Geometry check sheet. Reference: the model listing, model coordinates, mm. Face numbers are marked on the shaded views. A direction names the side the tool comes from. Coordinates: 2 decimals unless noted, no trailing zeros. Order: outer loops, then holes, each group sorted by start corner. A loop starts at its lowest first (then second) coordinate and runs counter-clockwise, first axis right, second up. Notation, with made-up numbers: (42, 19) -> (63, 19) arc R28 cw to (63, 52) -> close; hole circle Ø6 at (50.25, 70). An arc over 180 degrees is marked (long way). Answer as CSV lines item,"result". Start each with the question number.
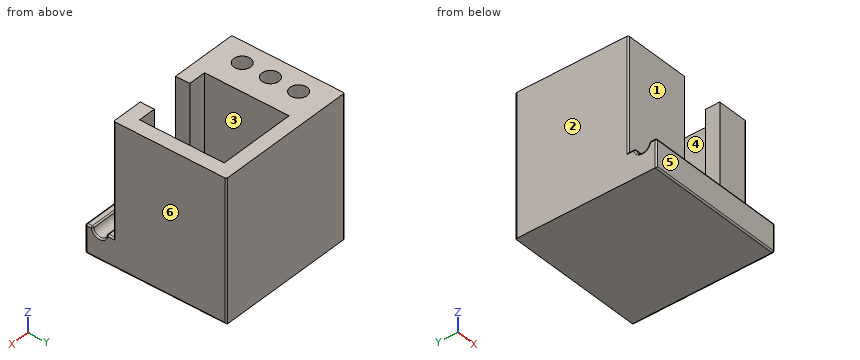
from build123d import *

# Parameters (mm, degrees)
F0_W     = 100
F0_H     = 100
F1_DEPTH = 100
F2_W     = 100
F2_H     = 20
F3_DEPTH = 80
F4_W     = 30
F4_H     = 10
F5_DEPTH = 80
F6_R     = 6
F7_DEPTH = 80
F9_DEPTH = 100
F10_R    = 1


with BuildPart() as f1:
    # F0 (on Top) → F1 (new body)
    with BuildSketch(Plane.XY):
        Rectangle(F0_W, F0_H)
    extrude(amount=F1_DEPTH)

    # F2 (on face) → F3 (cut)
    with BuildSketch(Plane.XY.offset(100)):
        with Locations((0, -40)):
            Rectangle(F2_W, F2_H)
    extrude(amount=-F3_DEPTH, mode=Mode.SUBTRACT)

    # F4 (on face) → F5 (cut, through all)
    with BuildSketch(Plane.XY.offset(100)):
        Polygon((40, 40), (-15, 40), (-15, -20), (-2.5, -20), (27.5, -20), (40, -20), align=None)
        with Locations((12.5, -25)):
            Rectangle(F4_W, F4_H)
    extrude(amount=-F5_DEPTH, mode=Mode.SUBTRACT)

    # F6 (on face) → F7 (cut, through all)
    with BuildSketch(Plane.XY.offset(100)):
        with Locations((-35, -10)):
            Circle(F6_R)
        with Locations((-35, 10)):
            Circle(F6_R)
        with Locations((-35, 30)):
            Circle(F6_R)
    extrude(amount=-F7_DEPTH, mode=Mode.SUBTRACT)

    # F8 (on face) → F9 (cut, through all)
    with BuildSketch(Plane.YZ.offset(50)):
        with BuildLine():
            ThreePointArc((-45, 20), (-40, 15), (-35, 20))
            Line((-35, 20), (-45, 20))
        make_face()
    extrude(amount=-F9_DEPTH, mode=Mode.SUBTRACT)

    # F10
    f10_edges = [f1.edges().sort_by_distance(p)[0] for p in [
        (0, -35, 20),
        (0, -45, 20),
        (50, -50, 10),
        (0, -50, 20),
        (-50, -50, 10),
        (0, -50, 0),
        (50, 0, 0),
        (50, -40, 15),
        (50, -47.5, 20),
        (50, -32.5, 20),
        (50, -30, 60),
        (-50, -40, 15),
        (-50, -47.5, 20),
        (-50, -32.5, 20),
        (50, 50, 50),
        (-50, -30, 60),
        (-50, 50, 50),
    ]]
    fillet(f10_edges, radius=F10_R)


solid = f1.part
Q1. Release check for a two-part mould opening along X. For the marked faces 3, 4, 5 and 6 record: released by +X, released by -X, zero draft, split by the parting line, or undercut.
Q2. Sectioned sample at C-C, the plane x = -35. Record the cut outline in (y, z).
Q3. Thickness scan on L1, parallel to Y at x = -35, z = 47; L2, parallel to X at y = 8.5, z = 22; L3, parallel to Y at x = -8.5, z = 84.5. Record the ranges inside material, lowest first.
Q4. Sectioned sample at D-D, the plane y = -25.5. Record the cut outline in (x, z).
Q5. Sectioned sample at B-B, the plane z = 37. Record the cut outline in (x, y), then the cut area to 3 significant figures.
Q6. Access from +Z, -Z, +X, -X, +Y, -Y to the whole of each face (thin tool, end or side, straight path). Record for the marked faces 1 and 2.
Q7. Go/stop test with flat-tipped pins: pin 1 Ø1 at (x, y) = (20, 30) entering from +Z; pin 2 Ø12 at (x, y) = (5.5, -10) entering from -Z; pin 3 Ø11 at (x, z) = (33.5, 64.5) entering from -Y; pin 4 Ø4 at (y, z) = (-33, 25.5) entering from -X. Record where each tip stops, or that it passes through.
Q8. Sectioned sample at A-A, the plane y = 37.5. Record the cut outline in (x, z), then the cut area to 3 significant figures.
Geometry results:
1,face 3,"undercut"
1,face 4,"undercut"
1,face 5,"zero draft"
1,face 6,"released by +X"
2,outline,"(-50, 1) arc R1 ccw to (-49, 0) -> (50, 0) -> (50, 100) -> (36, 100) -> (36, 20) -> (24, 20) -> (24, 100) -> (16, 100) -> (16, 20) -> (4, 20) -> (4, 100) -> (-4, 100) -> (-4, 20) -> (-16, 20) -> (-16, 100) -> (-30, 100) -> (-30, 20) -> (-34.08, 20) arc R1 ccw to (-35.07, 19.17) arc R5 cw to (-44.93, 19.17) arc R1 ccw to (-45.92, 20) -> (-49, 20) arc R1 ccw to (-50, 19) -> close"
3,L1,"y = -30 to -16, -4 to 4, 16 to 24, 36 to 50"
3,L2,"x = -50 to -40.81, -29.19 to -15, 40 to 50"
3,L3,"y = -30 to -20, 40 to 50"
4,outline,"(-50, 0) -> (49, 0) arc R1 ccw to (50, 1) -> (50, 100) -> (27.5, 100) -> (27.5, 20) -> (-2.5, 20) -> (-2.5, 100) -> (-50, 100) -> close"
5,outline,"(-50, -29) arc R1 ccw to (-49, -30) -> (-2.5, -30) -> (-2.5, -20) -> (-15, -20) -> (-15, 40) -> (40, 40) -> (40, -20) -> (27.5, -20) -> (27.5, -30) -> (49, -30) arc R1 ccw to (50, -29) -> (50, 49) arc R1 ccw to (49, 50) -> (-49, 50) arc R1 ccw to (-50, 49) -> close; hole circle Ø12 at (-35, -10); hole circle Ø12 at (-35, 10); hole circle Ø12 at (-35, 30)"
5,area,"4,060 mm^2"
6,face 1,"+Z, +X, -X, -Y"
6,face 2,"+Z, -Z, -X, +Y, -Y"
7,pin 1,"stops at z = 20"
7,pin 2,"stops at z = 0"
7,pin 3,"stops at y = -30"
7,pin 4,"passes through"
8,outline,"(-50, 0) -> (49, 0) arc R1 ccw to (50, 1) -> (50, 100) -> (40, 100) -> (40, 20) -> (-15, 20) -> (-15, 100) -> (-50, 100) -> close"
8,area,"5,600 mm^2"
